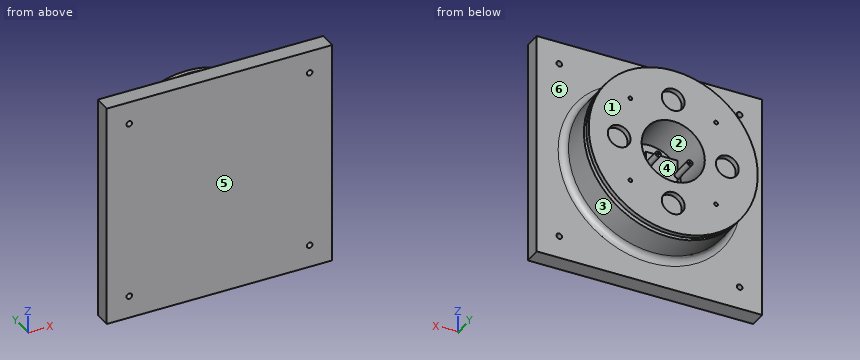
from build123d import *

# Parameters (mm, degrees)
SKETCH1_W                   = 200
SKETCH1_H                   = 200
BOSS_EXTRUDE1_DEPTH         = 15
SKETCH2_R                   = 2.5
BOSS_EXTRUDE2_DEPTH         = 31
SKETCH4_W                   = 28
SKETCH4_H                   = 28
BOSS_EXTRUDE3_DEPTH         = 10
LPATTERN2_COUNT             = 2
LPATTERN2_PITCH             = 28
FILLET1_R                   = 4
SKETCH8_R                   = 75
SKETCH8_R_2                 = 28
BOSS_EXTRUDE5_DEPTH         = 32
FILLET2_R                   = 6
SKETCH10_R                  = 67
SKETCH10_R_2                = 28
BOSS_EXTRUDE6_DEPTH         = 4
SKETCH11_R                  = 75
SKETCH11_R_2                = 28
BOSS_EXTRUDE7_DEPTH         = 4
SKETCH9_R                   = 10.1
CUT_EXTRUDE2_DEPTH          = 287.721118859
CIRPATTERN1_COUNT           = 4
SKETCH12_R                  = 10.1
BOSS_EXTRUDE8_DEPTH         = 3
CIRPATTERN2_COUNT           = 4
TAP_DRILL_FOR_M6X1_0_TAP1_D = 5
CIRPATTERN4_COUNT           = 4
CIRPATTERN5_COUNT           = 4
LPATTERN3_COUNT             = 2
LPATTERN3_PITCH             = 28


with BuildPart() as part:
    # Sketch1 → Boss-Extrude1 (new body)
    with BuildSketch(Plane(origin=(0, 0, 0), x_dir=(1, 0, 0), z_dir=(0, 1, 0))):
        with Locations((100, 100)):
            Rectangle(SKETCH1_W, SKETCH1_H)
    extrude(amount=BOSS_EXTRUDE1_DEPTH)

    # Sketch2 → Boss-Extrude2 (add)
    with BuildSketch(Plane(origin=(0, 15, 0), x_dir=(1, 0, 0), z_dir=(0, 1, 0))):
        with Locations(Location((80.5, 100, 0), (0, 0, 90))):
            Circle(SKETCH2_R)
    boss_extrude2 = extrude(amount=BOSS_EXTRUDE2_DEPTH)

    # Sketch4 → Boss-Extrude3 (add)
    with BuildSketch(Plane(origin=(0, 15, 0), x_dir=(1, 0, 0), z_dir=(0, 1, 0))):
        with Locations((94.5, 100)):
            Rectangle(SKETCH4_W, SKETCH4_H)
    extrude(amount=BOSS_EXTRUDE3_DEPTH)

    # LPattern2: Boss-Extrude2 ×2
    with Locations(*[(i * LPATTERN2_PITCH, 0, 0) for i in range(1, LPATTERN2_COUNT)]):
        add(boss_extrude2)

    # Fillet1
    fillet1_edges = [part.edges().sort_by_distance(p)[0] for p in [
        (78, 15, -100),
        (80.5, 15, -91.75),
        (80.5, 15, -108.25),
        (94.5, 15, -86),
        (108.5, 15, -91.75),
        (94.5, 15, -114),
        (108.5, 15, -108.25),
        (111, 15, -100),
    ]]
    fillet(fillet1_edges, radius=FILLET1_R)

    # Sketch8 → Boss-Extrude5 (add)
    with BuildSketch(Plane(origin=(0, 15, 0), x_dir=(1, 0, 0), z_dir=(0, 1, 0))):
        with Locations(Location((100, 100, 0), (0, 0, 90))):
            Circle(SKETCH8_R)
        with Locations(Location((100, 100, 0), (0, 0, 139.994799115))):
            Circle(SKETCH8_R_2, mode=Mode.SUBTRACT)
    extrude(amount=BOSS_EXTRUDE5_DEPTH)

    # Fillet2
    fillet2_edges = [part.edges().sort_by_distance(p)[0] for p in [
        (100, 15, -25),
    ]]
    fillet(fillet2_edges, radius=FILLET2_R)

    # Sketch10 → Boss-Extrude6 (add)
    with BuildSketch(Plane(origin=(0, 47, 0), x_dir=(1, 0, 0), z_dir=(0, 1, 0))):
        with Locations(Location((100, 100, 0), (0, 0, 270))):
            Circle(SKETCH10_R)
        with Locations(Location((100, 100, 0), (0, 0, 139.994799115))):
            Circle(SKETCH10_R_2, mode=Mode.SUBTRACT)
    extrude(amount=BOSS_EXTRUDE6_DEPTH)

    # Sketch11 → Boss-Extrude7 (add)
    with BuildSketch(Plane(origin=(0, 51, 0), x_dir=(1, 0, 0), z_dir=(0, 1, 0))):
        with Locations(Location((100, 100, 0), (0, 0, 90))):
            Circle(SKETCH11_R)
        with Locations(Location((100, 100, 0), (0, 0, 139.994799115))):
            Circle(SKETCH11_R_2, mode=Mode.SUBTRACT)
    extrude(amount=BOSS_EXTRUDE7_DEPTH)

    # Sketch9 → Cut-Extrude2 (cut, through all)
    with BuildSketch(Plane(origin=(0, 47, 0), x_dir=(1, 0, 0), z_dir=(0, 1, 0))):
        with Locations(Location((100, 148, 0), (0, 0, 270))):
            Circle(SKETCH9_R)
    cut_extrude2 = extrude(amount=CUT_EXTRUDE2_DEPTH, mode=Mode.SUBTRACT)

    # CirPattern1: Cut-Extrude2 ×4 about axis
    cirpattern1_axis = Axis((100, 0, -100), (0, 1, 0))
    for i in range(1, CIRPATTERN1_COUNT):
        add(cut_extrude2.rotate(cirpattern1_axis, i * 360 / CIRPATTERN1_COUNT), mode=Mode.SUBTRACT)

    # Sketch12 → Boss-Extrude8 (add)
    with BuildSketch(Plane(origin=(0, 47, 0), x_dir=(1, 0, 0), z_dir=(0, 1, 0))):
        with Locations(Location((100, 148, 0), (0, 0, 270))):
            Circle(SKETCH12_R)
    boss_extrude8 = extrude(amount=BOSS_EXTRUDE8_DEPTH)

    # CirPattern2: Boss-Extrude8 ×4 about axis
    cirpattern2_axis = Axis((100, 0, -100), (0, -1, 0))
    for i in range(1, CIRPATTERN2_COUNT):
        add(boss_extrude8.rotate(cirpattern2_axis, i * 360 / CIRPATTERN2_COUNT))

    # Tap Drill for M6x1.0 Tap1 (through all)
    with Locations(Plane(origin=(0, 15, 0), x_dir=(1, 0, 0), z_dir=(0, 1, 0))):
        with Locations((20, 20)):
            tap_drill_for_m6x1_0_tap1 = Hole(TAP_DRILL_FOR_M6X1_0_TAP1_D / 2)

    # CirPattern4: Tap Drill for M6x1.0 Tap1 ×4 about axis
    cirpattern4_axis = Axis((100, 0, -100), (0, 1, 0))
    for i in range(1, CIRPATTERN4_COUNT):
        add(tap_drill_for_m6x1_0_tap1.rotate(cirpattern4_axis, i * 360 / CIRPATTERN4_COUNT), mode=Mode.SUBTRACT)

    # Sketch23 → Tap Drill for M4x0.7 Tap2 (revolve, cut)
    with BuildSketch(Plane(origin=(138, 55, -138), x_dir=(0, 0, 1), z_dir=(1, 0, 0))):
        Polygon((0, 0), (0, 20.991420021), (1.65, 20), (1.65, 0), align=None)
    tap_drill_for_m4x0_7_tap2 = revolve(axis=Axis((138, 61.35, -138), (0, -1, 0)), mode=Mode.SUBTRACT)

    # CirPattern5: Tap Drill for M4x0.7 Tap2 ×4 about axis
    cirpattern5_axis = Axis((100, 0, -100), (0, 1, 0))
    for i in range(1, CIRPATTERN5_COUNT):
        add(tap_drill_for_m4x0_7_tap2.rotate(cirpattern5_axis, i * 360 / CIRPATTERN5_COUNT), mode=Mode.SUBTRACT)

    # Sketch28 → Tap Drill for M2x0.4 Tap1 (revolve, cut)
    with BuildSketch(Plane(origin=(80.5, 46, -100), x_dir=(0, 0, 1), z_dir=(1, 0, 0))):
        Polygon((0, 0), (0, 10.480688495), (0.8, 10), (0.8, 0), align=None)
    tap_drill_for_m2x0_4_tap1 = revolve(axis=Axis((80.5, 52.35, -100), (0, -1, 0)), mode=Mode.SUBTRACT)

    # LPattern3: Tap Drill for M2x0.4 Tap1 ×2
    with Locations(*[(i * LPATTERN3_PITCH, 0, 0) for i in range(1, LPATTERN3_COUNT)]):
        add(tap_drill_for_m2x0_4_tap1, mode=Mode.SUBTRACT)


solid = part.part
Input: part model. Units: mm. Frame: model coordinates. Face numbers are marked on the shaded views. A direction names the side the tool comes from. Coordinates: 2 decimals unless noted, no trailing zeros. Write item = value, one per line. Start each with the question number.
(1) Line query: line 1 along Y through (x, z) = (19, -79); line 2 along Y through (x, z) = (163.5, -63.5); line 3 along X through (y, z) = (41, -138). Output: solid intervals per line, ascending. Write a range as [from, to].
(2) Pull-direction query (X, two-part tool) for the marked faces 1, 2, 3 and 4; classes: released by +X, released by -X, zero draft, split by the parting line, or undercut.
(3) Section A-A on y = 38.5. Give the number of separate pieces and of enclosed holes in the cut face, and give its area (3 significant figures).
(4) First-contact query: P1, Ø10, axis at y = 25.5, z = -128, coming from the +X side; P2, Ø12, axis at y = 48.5, z = -94.5, coming from the -X side; P3, Ø6.5, axis at x = 95.5, y = 22, coming from the +Z side. Flat tips, straight axial feed; report the tip coordinate or a pass-through.
(5) Reachability of the marked faces 5 and 6 from +Z, -Z, +X, -X, +Y, -Y: full face, straight path, thin tool, end or side. Return the list, or none.
Result set:
q1.line_1 = [0, 15]
q1.line_2 = [0, 47], [51, 55]
q1.line_3 = [35.34, 60.35], [63.65, 136.35], [139.65, 164.66]
q2.face_1 = zero draft
q2.face_2 = undercut
q2.face_3 = split by the parting line
q2.face_4 = undercut
q3.separate_pieces = 3
q3.enclosed_holes = 7
q3.area = 15,200 mm²
q4.P1 = 171.39
q4.P2 = 25
q4.P3 = -24.68
q5.face_5 = +Z, -Z, +X, -X, -Y
q5.face_6 = +Y
